from build123d import *

# Parameters (mm, degrees)
FILLET1_R      = 0.1
FILLET2_R      = 0.12
CHAMFER1_SIZE  = 0.2
EXTRUDE1_DEPTH = 1


with BuildPart() as part:
    # Sketch1 → Revolve1 (revolve)
    with BuildSketch(Plane.XY, mode=Mode.PRIVATE) as revolve1_sk:
        Polygon((2, 1), (2, 0), (4.279914881, 0), (8, 0), (8, 1), align=None)
        Polygon((0, 1.9), (0, 0), (2, 0), (2, 1), (2, 1.9), align=None)
    revolve(revolve1_sk.sketch.rotate(Axis((0, 0, 0), (1, 0, 0)), 90), axis=Axis((0, 0, 0), (1, 0, 0)))

    # Fillet1
    fillet1_edges = [part.edges().sort_by_distance(p)[0] for p in [
        (2, 0, -1),
    ]]
    fillet(fillet1_edges, radius=FILLET1_R)

    # Fillet2
    fillet2_edges = [part.edges().sort_by_distance(p)[0] for p in [
        (0, 0, -1.9),
    ]]
    fillet(fillet2_edges, radius=FILLET2_R)

    # Chamfer1
    chamfer1_edges = [part.edges().sort_by_distance(p)[0] for p in [
        (8, 0, -1),
    ]]
    chamfer(chamfer1_edges, length=CHAMFER1_SIZE)

    # Sketch2 → Extrude1 (cut)
    with BuildSketch(Plane.ZY):
        Polygon((0, 0.866025404), (-0.75, 0.433012702), (-0.75, -0.433012702), (0, -0.866025404), (0.75, -0.433012702), (0.75, 0.433012702), align=None)
    extrude(amount=-EXTRUDE1_DEPTH, mode=Mode.SUBTRACT)


solid = part.part
Input: part model. Units: mm. Frame: model coordinates. A direction names the side the tool comes from. Give positions to 0.01 mm unless a question says otherwise; leave off trailing zeros. Write each loop counter-clockwise with the first axis right and the second up, starting at its lowest first coordinate (ties: lowest second). Pieces come first, ordered by that corner, then holes. Notation, with made-up numbers: M 62,-32 L 101,-32 A24 cw 101,-2 Z; hole C 88,-35 d5. An arc over 180 degrees is marked long. Write item = value, one per line. Start each with the question number.
1) Cut plane B-B on x = 2.25. Return the cut outline in (y, z), then the cut area to 3 significant figures.
2) Material intervals for line 1 along Z through (x, y) = (2.75, -0.9); line 2 along X through (y, z) = (-1.5, 0.5); line 3 along X through (y, z) = (0.45, 0.4), sorted ascending. Write a range as [from, to].
3) Reachability of faces 1 (the flat face through (2, 1, -1)), 2 (the flat face through (0, 0, 1)), 3 (the flat face through (1, 0, 0)) from +Z, -Z, +X, -X, +Y, -Y: full face, straight path, thin tool, end or side. Return the list, or none.
4) Cut plane A-A on y = 0. Return the cut outline in (x, z).
5) Draft query along Y for faces 4 (the flat face through (8, 0, 0)), 5 (the flat face through (0.5, 0, -0.75)), 6 (the cylindrical face through (5, 1, 0)). Return one class per face: +Y half, -Y half, draft (parallel to the pull), parting line (faces both ways), or undercut.
Solved:
q1.outline = C 0,0 d2
q1.area = 3.14 mm2
q2.line_1 = [-0.44, 0.44]
q2.line_2 = [0, 2]
q2.line_3 = [1, 8]
q3.face_1 = +X
q3.face_2 = +Z, -Z, -X, +Y, -Y
q3.face_3 = -X
q4.outline = M 0,-1.78 A0.12 ccw 0.12,-1.9 L 2,-1.9 L 2,-1.1 A0.1 cw 2.1,-1 L 7.8,-1 L 8,-0.8 L 8,0.8 L 7.8,1 L 2.1,1 A0.1 cw 2,1.1 L 2,1.9 L 0.12,1.9 A0.12 ccw 0,1.78 L 0,0.75 L 1,0.75 L 1,-0.75 L 0,-0.75 Z
q5.face_4 = draft
q5.face_5 = undercut
q5.face_6 = parting line
